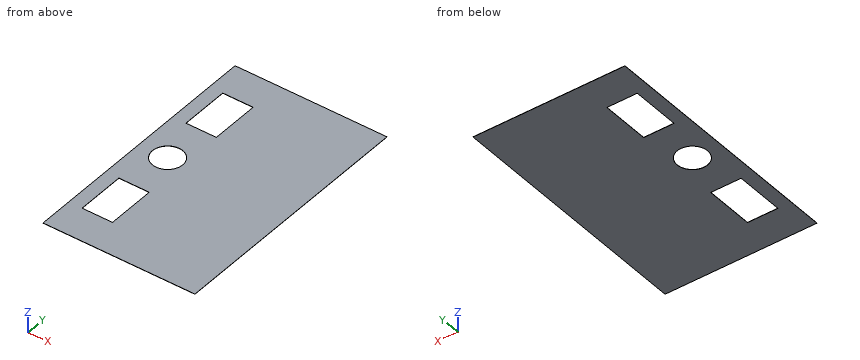
```python
from build123d import *

# Parameters (mm, degrees)
F0_W     = 1250
F0_H     = 2090
F0_W_2   = 250
F0_H_2   = 400
F0_R     = 125
F1_DEPTH = 1.6


with BuildPart() as f1:
    # F0 (on Top) → F1 (new body)
    with BuildSketch(Plane.XY):
        Rectangle(F0_W, F0_H)
        with Locations((-390, -565)):
            Rectangle(F0_W_2, F0_H_2, mode=Mode.SUBTRACT)
        with Locations((-390, 0)):
            Circle(F0_R, mode=Mode.SUBTRACT)
        with Locations((-390, 565)):
            Rectangle(F0_W_2, F0_H_2, mode=Mode.SUBTRACT)
    extrude(amount=F1_DEPTH)


solid = f1.part
```
Part model, mm, in its own coordinate system. Coordinates: 2 decimals unless noted, no trailing zeros. Loops run counter-clockwise (first coordinate to the right, second up) from the corner with the lowest first, then second, coordinate; pieces in that order, holes last. Notation, with made-up numbers: (11.25, 8.25) - (55.25, 8.25) arc R14 cw to (55.25, 34.25) - close; hole circle Ø2 at (4.5, 63). An arc over 180 degrees is marked (long way). Write item = value, one per line. Start each with the question number.
Item 1: Wall check: L1, parallel to Y at x = -390, z = 1.1; L2, parallel to Y at x = -288.5, z = 0.85; L3, parallel to X at y = 22, z = 0.4. Give the ranges that are in metal, low to high. Write a range as from..to.
Item 2: Flat gauge pin, fed straight in: pin 1 Ø10 at (x, y) = (-201, 22) entering from -Z. Where does the tip first touch, or does it go through?
Item 3: Cut at B-B, the plane z = 0.25. Give the cut face in (x, y), and give its area (3 significant figures).
Item 4: Cut at A-A, the plane y = 0. Give the cut face in (x, z).
Item 5: Cut at C-C, the plane x = -421.5. Give the cut face in (y, z), and give its area (3 significant figures).
The answers:
q1.L1 = -1045..-765, -365..-125, 125..365, 765..1045
q1.L2 = -1045..-765, -365..-72.96, 72.96..365, 765..1045
q1.L3 = -625..-513.05, -266.95..625
q2.pin_1 = 0
q3.outline = (-625, -1045) - (625, -1045) - (625, 1045) - (-625, 1045) - close; hole (-515, -765) - (-265, -765) - (-265, -365) - (-515, -365) - close; hole circle Ø250 at (-390, 0); hole (-515, 365) - (-265, 365) - (-265, 765) - (-515, 765) - close
q3.area = 2,360,000 mm2
q4.outline = (-625, 0) - (-515, 0) - (-515, 1.6) - (-625, 1.6) - close; (-265, 0) - (625, 0) - (625, 1.6) - (-265, 1.6) - close
q5.outline = (-1045, 0) - (-765, 0) - (-765, 1.6) - (-1045, 1.6) - close; (-365, 0) - (-120.97, 0) - (-120.97, 1.6) - (-365, 1.6) - close; (120.97, 0) - (365, 0) - (365, 1.6) - (120.97, 1.6) - close; (765, 0) - (1045, 0) - (1045, 1.6) - (765, 1.6) - close
q5.area = 1,680 mm2
